Read the model definition and answer for the solid it produces. Units are mm, in the model's axes. Coordinates: 2 decimals unless noted, no trailing zeros. Loops run counter-clockwise (first coordinate to the right, second up) from the corner with the lowest first, then second, coordinate; pieces in that order, holes last. Notation, with made-up numbers: (4, -20) - (62, -20) arc R27 cw to (62, -2) - close; hole circle Ø7 at (69.5, 1). An arc over 180 degrees is marked (long way). Use one line per item in the form item = value. Start each with the question number.
1) A cutting plane is placed at A-A (z = 26). Give the vertices of the cut face in (x, y) (3 decimals).
2) Each of these flat-tipped pins is pushed along its axis until it touches: P1, Ø1, axis at x = -2.5, z = -29, coming from the +Y side; P2, Ø0.6, axis at x = 10, y = 1, coming from the -Z side. Where does it stop, or does it pass through?
3) Consider line 1 (X direction, y = 1.1, z = 35) (3 decimals); line 2 (X direction, y = 2.55, z = 28.5) (3 decimals); line 3 (Z direction, x = 5, y = 0.95). Determine where each line is inside the solid, lowest interval first.
4) A cutting plane is placed at C-C (y = 0.6). State how many separate pieces and enclosed holes the cut face has, and give its area (3 significant figures).
5) A cutting plane is placed at B-B (x = -4.5). Give the vertices of the cut face in (y, z) (3 decimals).
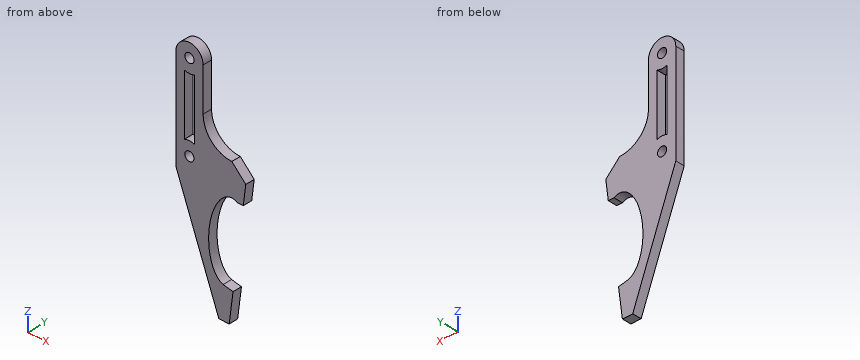
from build123d import *

# Parameters (mm, degrees)
CROQUIS1_R                   = 1.5875
SALIENTE_EXTRUIR1_DEPTH      = 3.175
CORTAR_EXTRUIR1_DEPTH        = 3.175
CORTAR_EXTRUIR3_DEPTH        = 10
CROQUIS4_R                   = 10
CORTAR_EXTRUIR4_DEPTH        = 10
REDONDEO1_R                  = 2
ENL_V_MAT_EXTRU_1_DEPTH      = 43.027736377
ENL_V_MAT_EXTRU_1_DEPTH_BACK = 4
ESQUISSE1_RX                 = 14
ESQUISSE1_RY                 = 7.031711939
ESQUISSE2_W                  = 9.071953096
ESQUISSE2_H                  = 3.948156649
ENL_V_MAT_EXTRU_2_DEPTH      = 43.02773651
CHANFREIN1_START             = -27.627623392
CHANFREIN1_OUTLINE_W         = 3.506874848
CHANFREIN1_OUTLINE_H         = 3.175
CHANFREIN1_DEPTH             = 1.390086692
CHANFREIN1_START_2           = -27.652783734
CHANFREIN1_2_OUTLINE_W       = 3.506874848
CHANFREIN1_2_OUTLINE_H       = 3.175
CHANFREIN1_2_DEPTH           = 0.025160342


with BuildPart() as part:
    # Croquis1 → Saliente-Extruir1 (new body)
    with BuildSketch(Plane(origin=(0, 0, 0), x_dir=(1, 0, 0), z_dir=(0, 1, 0))):
        with BuildLine():
            Line((-12.5, 0), (-12.5, -40))
            Line((-12.5, -40), (-2.975, -40))
            Line((-2.975, -40), (-2.975, -20))
            ThreePointArc((-2.975, -20), (-0.046067812, -12.928932188), (7.025, -10))
            Line((7.025, -10), (12.5, -10))
            Line((12.5, -10), (12.5, 40))
            Line((12.5, 40), (2.5, 40))
            Line((2.5, 40), (-12.5, 0))
        make_face()
        with Locations(Location((-7.7375, -5, 0), (0, 0, 270))):
            Circle(CROQUIS1_R, mode=Mode.SUBTRACT)
        with Locations(Location((-7.7375, -35, 0), (0, 0, 270))):
            Circle(CROQUIS1_R, mode=Mode.SUBTRACT)
    extrude(amount=SALIENTE_EXTRUIR1_DEPTH)

    # Croquis2 → Cortar-Extruir1 (cut)
    with BuildSketch(Plane(origin=(0, 3.175, 0), x_dir=(1, 0, 0), z_dir=(0, 1, 0))):
        Polygon((12.5, -10), (6.1, 40), (12.5, 40), align=None)
    extrude(amount=-CORTAR_EXTRUIR1_DEPTH, mode=Mode.SUBTRACT)

    # Croquis3 → Cortar-Extruir3 (cut)
    with BuildSketch(Plane(origin=(0, 3.175, 0), x_dir=(1, 0, 0), z_dir=(0, 1, 0))):
        with BuildLine():
            ThreePointArc((-5.975, -30.575635639), (-7.7375, -30.2375), (-9.5, -30.575635639))
            Line((-9.5, -30.575635639), (-9.5, -9.427055314))
            ThreePointArc((-9.5, -9.427055314), (-7.7375, -9.765), (-5.975, -9.427055314))
            Line((-5.975, -9.427055314), (-5.975, -14.803847577))
            Line((-5.975, -14.803847577), (-5.975, -30.575635639))
        make_face()
        with BuildLine():
            ThreePointArc((-12.5, -35), (-7.7375, -39.7625), (-2.975, -35))
            Line((-2.975, -35), (-2.975, -40))
            Line((-2.975, -40), (-12.5, -40))
            Line((-12.5, -40), (-12.5, -35))
        make_face()
    extrude(amount=-CORTAR_EXTRUIR3_DEPTH, mode=Mode.SUBTRACT)

    # Croquis4 → Cortar-Extruir4 (cut)
    with BuildSketch(Plane(origin=(0, 3.175, 0), x_dir=(1, 0, 0), z_dir=(0, 1, 0))):
        with Locations((9.274103387, 15.202317292)):
            Circle(CROQUIS4_R)
        Polygon((7.025, -10), (11.878723404, -5.146276596), (12.5, -10), align=None)
    extrude(amount=-CORTAR_EXTRUIR4_DEPTH, mode=Mode.SUBTRACT)

    # Redondeo1
    redondeo1_edges = [part.edges().sort_by_distance(p)[0] for p in [
        (8.004462032, 1.5875, -25.121390375),
        (10.543744741, 1.5875, -5.283244209),
    ]]
    fillet(redondeo1_edges, radius=REDONDEO1_R)

    # Esquisse1 → Enlèv. mat.-Extru.1 (cut, two sides: drawn at the far end of the back side and taken through both)
    with BuildSketch(Plane.XZ.offset(-ENL_V_MAT_EXTRU_1_DEPTH_BACK)):
        with Locations(Location((6.06176106, -15.09925225), (0, 0, -95.443545347))):
            Ellipse(ESQUISSE1_RX, ESQUISSE1_RY)
    extrude(amount=ENL_V_MAT_EXTRU_1_DEPTH + ENL_V_MAT_EXTRU_1_DEPTH_BACK, mode=Mode.SUBTRACT)

    # Esquisse2 → Enlèv. mat.-Extru.2 (cut, through all)
    with BuildSketch(Plane(origin=(0, 3.175, 0), x_dir=(1, 0, 0), z_dir=(0, 1, 0))):
        with Locations((11.233998337, 3.697201044)):
            Rectangle(ESQUISSE2_W, ESQUISSE2_H)
    extrude(amount=-ENL_V_MAT_EXTRU_2_DEPTH, mode=Mode.SUBTRACT)

    # Chanfrein1: read off the stored shape, not the designer's step
    # Chanfrein1 outline → Chanfrein1 (cut)
    with BuildSketch(Plane(origin=(0, 0, 0), x_dir=(0.9823357851879482, 0, -0.18712670878091503), z_dir=(0.18712670878091503, 0, 0.9823357851879482)).offset(CHANFREIN1_START)):
        with Locations((11.081851268, 1.5875)):
            Rectangle(CHANFREIN1_OUTLINE_W, CHANFREIN1_OUTLINE_H)
    extrude(amount=CHANFREIN1_DEPTH, mode=Mode.SUBTRACT)

    # Chanfrein1 2 outline → Chanfrein1 2 (add)
    with BuildSketch(Plane(origin=(0, 0, 0), x_dir=(0.9823357851879482, 0, -0.18712670878091503), z_dir=(0.18712670878091503, 0, 0.9823357851879482)).offset(CHANFREIN1_START_2)):
        with Locations((11.081851268, 1.5875)):
            Rectangle(CHANFREIN1_2_OUTLINE_W, CHANFREIN1_2_OUTLINE_H)
    extrude(amount=CHANFREIN1_2_DEPTH)


solid = part.part
Found:
q1.outline = (-12.5, 0) - (-9.5, 0) - (-9.5, 3.175) - (-12.5, 3.175) - close; (-5.975, 0) - (-2.975, 0) - (-2.975, 3.175) - (-5.975, 3.175) - close
q2.P1 = through
q2.P2 = -1.72
q3.line_1 = -12.5 to -9.325, -6.15 to -2.975
q3.line_2 = -12.5 to -9.5, -5.975 to -2.975
q3.line_3 = -40 to -29.08, -1.73 to 10.21
q4.separate_pieces = 1
q4.enclosed_holes = 3
q4.area = 739 mm^2
q5.outline = (0, -21.333) - (3.175, -21.333) - (3.175, 38.493) - (0, 38.493) - close
